from build123d import *

# Parameters (mm, degrees)
SKETCH1_R             = 15
SKETCH1_R_2           = 1.8288
SKETCH1_R_3           = 11.1125
BOSS_EXTRUDE1_DEPTH   = 3.175
CUT_EXTRUDE1_REACH    = 173.858
SKETCH2_W             = 4.112404804
SKETCH2_H             = 127.6975
FILLET3_R             = 2.5
FILLET4_R             = 25
F_6_CLEARANCE_HOLE1_D = 3.7973


with BuildPart() as part:
    # Sketch1 → Boss-Extrude1 (new body)
    with BuildSketch(Plane(origin=(0, 0, 0), x_dir=(0, 0, -1), z_dir=(1, 0, 0))):
        with BuildLine():
            Line((20.757404804, -103.81), (20.757404804, -5))
            Line((20.757404804, -5), (16.645, 5.681808734))
            Line((16.645, 5.681808734), (16.645, 35))
            ThreePointArc((16.645, 35), (14.175569213, 43.724062271), (7.5, 49.85954323))
            Line((7.5, 49.85954323), (7.5, 121.151519965))
            ThreePointArc((7.5, 121.151519965), (0, 170), (-7.5, 121.151519965))
            Line((-7.5, 121.151519965), (-7.5, 49.85954323))
            ThreePointArc((-7.5, 49.85954323), (-14.175569213, 43.724062271), (-16.645, 35))
            Line((-16.645, 35), (-16.645, 5.681808734))
            Line((-16.645, 5.681808734), (-20.757404804, -5))
            Line((-20.757404804, -5), (-20.757404804, -103.81))
            Line((-20.757404804, -103.81), (20.757404804, -103.81))
        make_face()
        with Locations((0, 145)):
            Circle(SKETCH1_R, mode=Mode.SUBTRACT)
        with Locations((-13.4747, -100)):
            Circle(SKETCH1_R_2, mode=Mode.SUBTRACT)
        with Locations((13.4747, -100)):
            Circle(SKETCH1_R_2, mode=Mode.SUBTRACT)
        with Locations((-13.4747, 0)):
            Circle(SKETCH1_R_2, mode=Mode.SUBTRACT)
        with Locations((13.4747, 0)):
            Circle(SKETCH1_R_2, mode=Mode.SUBTRACT)
        with Locations((0, 35)):
            Circle(SKETCH1_R_3, mode=Mode.SUBTRACT)
    extrude(amount=BOSS_EXTRUDE1_DEPTH)

    # Sketch2 → Cut-Extrude1 (cut, up to next)
    with BuildSketch(Plane(origin=(3.175, 0, 0), x_dir=(0, 0, -1), z_dir=(1, 0, 0)), mode=Mode.PRIVATE) as cut_extrude1_sk1:
        Polygon((11.645, -5), (-11.645, -5), (11.645, -27.976379872), align=None)
    cut_extrude1_tool1 = extrude(cut_extrude1_sk1.sketch, amount=-CUT_EXTRUDE1_REACH, mode=Mode.PRIVATE) & part.part
    # Sketch2 → Cut-Extrude1 (cut, up to next)
    with BuildSketch(Plane(origin=(3.175, 0, 0), x_dir=(0, 0, -1), z_dir=(1, 0, 0)), mode=Mode.PRIVATE) as cut_extrude1_sk2:
        Polygon((-11.645, -12.023620128), (11.645, -35), (-11.645, -57.976379872), (-11.645, -35), align=None)
    cut_extrude1_tool2 = extrude(cut_extrude1_sk2.sketch, amount=-CUT_EXTRUDE1_REACH, mode=Mode.PRIVATE) & part.part
    # Sketch2 → Cut-Extrude1 (cut, up to next)
    with BuildSketch(Plane(origin=(3.175, 0, 0), x_dir=(0, 0, -1), z_dir=(1, 0, 0)), mode=Mode.PRIVATE) as cut_extrude1_sk3:
        Polygon((-11.645, -72.023620128), (-11.645, -95), (11.645, -95), align=None)
    cut_extrude1_tool3 = extrude(cut_extrude1_sk3.sketch, amount=-CUT_EXTRUDE1_REACH, mode=Mode.PRIVATE) & part.part
    # Sketch2 → Cut-Extrude1 (cut, up to next)
    with BuildSketch(Plane(origin=(3.175, 0, 0), x_dir=(0, 0, -1), z_dir=(1, 0, 0)), mode=Mode.PRIVATE) as cut_extrude1_sk4:
        Polygon((11.645, -42.023620128), (11.645, -65), (11.645, -87.976379872), (-11.645, -65), align=None)
    cut_extrude1_tool4 = extrude(cut_extrude1_sk4.sketch, amount=-CUT_EXTRUDE1_REACH, mode=Mode.PRIVATE) & part.part
    # Sketch2 → Cut-Extrude1 (cut, up to next)
    with BuildSketch(Plane(origin=(3.175, 0, 0), x_dir=(0, 0, -1), z_dir=(1, 0, 0)), mode=Mode.PRIVATE) as cut_extrude1_sk5:
        with Locations((-18.701202402, -39.96125)):
            Rectangle(SKETCH2_W, SKETCH2_H)
    cut_extrude1_tool5 = extrude(cut_extrude1_sk5.sketch, amount=-CUT_EXTRUDE1_REACH, mode=Mode.PRIVATE) & part.part
    # Sketch2 → Cut-Extrude1 (cut, up to next)
    with BuildSketch(Plane(origin=(3.175, 0, 0), x_dir=(0, 0, -1), z_dir=(1, 0, 0)), mode=Mode.PRIVATE) as cut_extrude1_sk6:
        with Locations((18.701202402, -39.96125)):
            Rectangle(SKETCH2_W, SKETCH2_H)
    cut_extrude1_tool6 = extrude(cut_extrude1_sk6.sketch, amount=-CUT_EXTRUDE1_REACH, mode=Mode.PRIVATE) & part.part
    add(cut_extrude1_tool1.solids().sort_by_distance((3.175, -12.658793, -3.881667))[0], mode=Mode.SUBTRACT)
    add(cut_extrude1_tool2.solids().sort_by_distance((3.175, -35, 3.881667))[0], mode=Mode.SUBTRACT)
    add(cut_extrude1_tool3.solids().sort_by_distance((3.175, -87.341207, 3.881667))[0], mode=Mode.SUBTRACT)
    add(cut_extrude1_tool4.solids().sort_by_distance((3.175, -65, -3.881667))[0], mode=Mode.SUBTRACT)
    add(cut_extrude1_tool5.solids().sort_by_distance((3.175, -39.96125, 18.701202))[0], mode=Mode.SUBTRACT)
    add(cut_extrude1_tool6.solids().sort_by_distance((3.175, -39.96125, -18.701202))[0], mode=Mode.SUBTRACT)

    # Fillet3
    fillet3_edges = [part.edges().sort_by_distance(p)[0] for p in [
        (1.5875, -103.81, 16.645),
        (1.5875, -12.023620128, 11.645),
        (1.5875, -35, -11.645),
        (1.5875, -57.976379872, 11.645),
        (1.5875, -103.81, -16.645),
        (1.5875, -72.023620128, 11.645),
        (1.5875, -95, -11.645),
        (1.5875, -95, 11.645),
        (1.5875, -87.976379872, -11.645),
        (1.5875, -65, 11.645),
        (1.5875, -42.023620128, -11.645),
        (1.5875, -27.976379872, -11.645),
        (1.5875, -5, 11.645),
        (1.5875, -5, -11.645),
    ]]
    fillet(fillet3_edges, radius=FILLET3_R)

    # Fillet4
    fillet4_edges = [part.edges().sort_by_distance(p)[0] for p in [
        (1.5875, 49.85954323, 7.5),
        (1.5875, 121.151519965, 7.5),
        (1.5875, 121.151519965, -7.5),
        (1.5875, 49.85954323, -7.5),
    ]]
    fillet(fillet4_edges, radius=FILLET4_R)

    # #6 Clearance Hole1 (through all)
    with Locations(Plane(origin=(3.175, 0, 0), x_dir=(0, 0, -1), z_dir=(1, 0, 0))):
        with Locations((0, 90)):
            Hole(F_6_CLEARANCE_HOLE1_D / 2)


solid = part.part
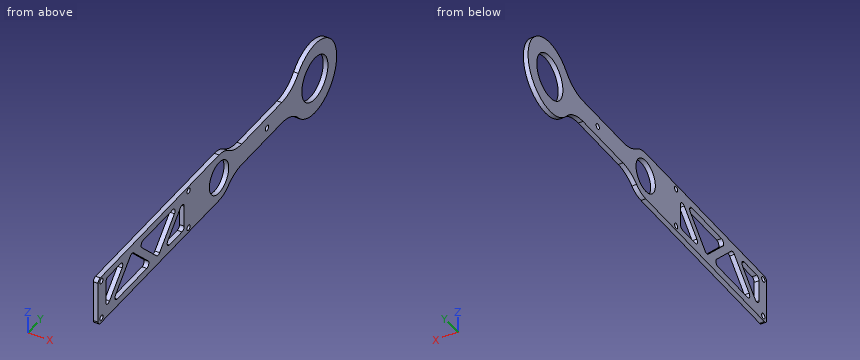
Geometry: final body of the model. Coordinates: model frame, mm. Give positions to 0.01 mm unless a question says otherwise; leave off trailing zeros. Order: outer loops, then holes, each group sorted by start corner. A loop starts at its lowest first (then second) coordinate and runs counter-clockwise, first axis right, second up. Notation, with made-up numbers: (-34.75, 33.5) -> (-14.75, 33.5) arc R21 cw to (-14.75, 46.5) -> close; hole circle Ø10 at (-7.75, 31). An arc over 180 degrees is marked (long way). Answer as a JSON object with one key per item and string values.
Q1. Material intervals for probe 1 along Z at (x, y) = (0.8, -100) (1 decimal); probe 2 along Z at (x, y) = (1.1, 90); probe 3 along Z at (x, y) = (1.65, 94), sorted ascending.
Entries:
{"probe 1": "z = -16.6 to -15.3, -11.6 to 11.6, 15.3 to 16.6", "probe 2": "z = -7.5 to -1.9, 1.9 to 7.5", "probe 3": "z = -7.5 to 7.5"}
Q2. First-contact query: pin 1 (4 mm diameter, centred on y = -100, z = -13.47, fed in from -X); pin 2 (1.6 mm diameter, centred on x = 2, y = 79.5, fed in from +Z); pin 3 (1 mm diameter, centred on x = 2, y = -83.5, fed in from -Z) (3 decimals); pin 4 (1.5 mm diameter, centred on x = 1.5, y = 129, fed in from -Z). Flat tips, straight axial feed; report the tip coordinate or a pass-through.
Entries:
{"pin 1": "stops at x = 0", "pin 2": "stops at z = 7.5", "pin 3": "stops at z = -16.645", "pin 4": "stops at z = -19.81"}
Q3. Section B-B (x = 1.65). State how many separate pieces and enclosed holes the cut face has, plus the area to 3 significant figures.
Entries:
{"separate pieces": "1", "enclosed holes": "11", "area": "5,450 mm^2"}
Q4. Section C-C (y = -41.5). Output: boundary loops of the cut face in (x, z) (3 decimals), plus the area to 3 significant figures.
Entries:
{"outline": "(0, -16.645) -> (3.175, -16.645) -> (3.175, -5.056) -> (0, -5.056) -> close; (0, 11.645) -> (3.175, 11.645) -> (3.175, 16.645) -> (0, 16.645) -> close", "area": "52.7 mm^2"}
Q5. Section D-D (y = 82). Output: boundary loops of the cut face in (x, z) (3 decimals).
Entries:
{"outline": "(0, -7.5) -> (3.175, -7.5) -> (3.175, 7.5) -> (0, 7.5) -> close"}
Q6. Section A-A (y = 145). Output: boundary loops of the cut face in (x, z) (3 decimals), plus the area to 3 significant figures.
Entries:
{"outline": "(0, -25) -> (3.175, -25) -> (3.175, -15) -> (0, -15) -> close; (0, 15) -> (3.175, 15) -> (3.175, 25) -> (0, 25) -> close", "area": "63.5 mm^2"}
